Could you check a few things on this drawing? It's one solid part, dimensions in mm from its lowest x, y, z. A direction names the side the tool comes from. Round coordinates to 2 decimals unless told otherwise and drop trailing zeros. Loops run counter-clockwise (first coordinate to the right, second up) from the corner with the lowest first, then second, coordinate; pieces in that order, holes last. Notation, with made-up numbers: M 22.25,7.5 L 42.25,7.5 A34 ccw 42.25,44.5 Z; hole C 60,3 d5. An arc over 180 degrees is marked long. Write item = value, one per line. Start each with the question number.
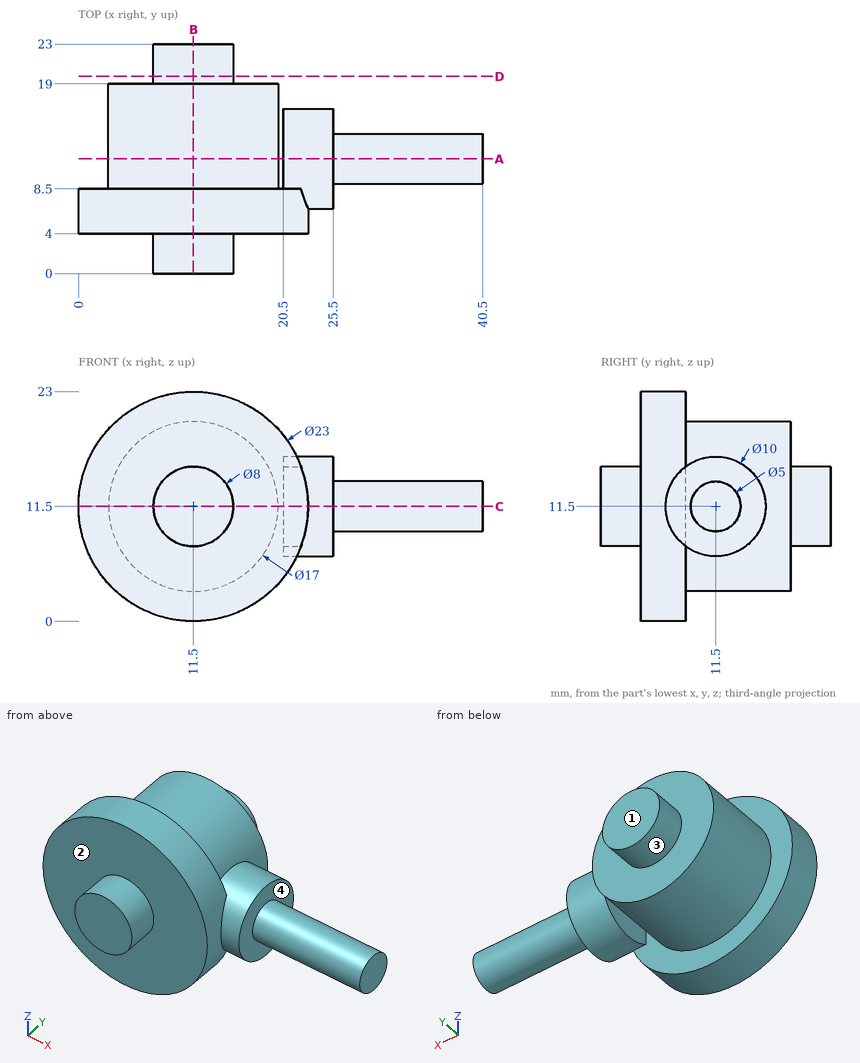
Item 1: I want a section at B-B, the plane x = 11.5. List the corners of the cut face in (y, z) for me, then the cut area to 3 significant figures.
Item 2: I want a section at D-D, the plane y = 19.75. List the corners of the cut face in (x, z) for me.
Item 3: Will these pins go through, and if not, where does the flat tip stop? pin 1 Ø8 at (x, z) = (34, 12.5) entering from -Y; pin 2 Ø10 at (x, z) = (8, 9.5) entering from +Y; pin 3 Ø1.5 at (x, z) = (35, 8) entering from +Y; pin 4 Ø5 at (y, z) = (17, 16.5) entering from -X.
Item 4: I want a section at C-C, the plane z = 11.5. List the corners of the cut face in (x, y) for me, then the cut area to 3 significant figures.
Item 5: Please list where these lines run through material, in increasing order: line 1 (Y direction, x = 12, z = 15.75); line 2 (X direction, y = 10, z = 15.25); line 3 (Y direction, x = 11.5, z = 21.25). Write a range as [from, to].
Item 6: I want a section at A-A, the plane y = 11.5. List the corners of the cut face in (x, z) for me, then the cut area to 3 significant figures.
Item 7: For the marked faces 1, 2, 3 and 4, which set-ups out of +Z, -Z, +X, -X, +Y, -Y let a thin tool reach every point of the face, with its end or its side?
Worked out:
q1.outline = M 0,7.5 L 4,7.5 L 4,0 L 8.5,0 L 8.5,3 L 19,3 L 19,7.5 L 23,7.5 L 23,15.5 L 19,15.5 L 19,20 L 8.5,20 L 8.5,23 L 4,23 L 4,15.5 L 0,15.5 Z
q1.area = 346 mm2
q2.outline = C 11.5,11.5 d8
q3.pin_1 = 9
q3.pin_2 = 23
q3.pin_3 = through
q3.pin_4 = 3.38
q4.outline = M 0,4 L 7.5,4 L 7.5,0 L 15.5,0 L 15.5,4 L 23,4 L 23,6.5 L 25.5,6.5 L 25.5,9 L 40.5,9 L 40.5,14 L 25.5,14 L 25.5,16.5 L 20.5,16.5 L 20.5,8.5 L 20,8.5 L 20,19 L 15.5,19 L 15.5,23 L 7.5,23 L 7.5,19 L 3,19 L 3,8.5 L 0,8.5 Z
q4.area = 466 mm2
q5.line_1 = [4, 19]
q5.line_2 = [3.87, 19.13], [20.5, 25.5]
q5.line_3 = [4, 8.5]
q6.outline = C 11.5,11.5 d17; M 20.5,6.5 L 25.5,6.5 L 25.5,9 L 40.5,9 L 40.5,14 L 25.5,14 L 25.5,16.5 L 20.5,16.5 Z
q6.area = 352 mm2
q7.face_1 = +Z, -Z, +X, -X, +Y
q7.face_2 = -Y
q7.face_3 = +Y
q7.face_4 = +X
